Model file for the job. Use its own axes, mm. Face numbers are marked on the shaded views. Give positions to 0.01 mm unless a question says otherwise; leave off trailing zeros. Loops run counter-clockwise (first coordinate to the right, second up) from the corner with the lowest first, then second, coordinate; pieces in that order, holes last. Notation, with made-up numbers: M 66,-35.75 L 100,-35.75 A12 cw 100,-31.75 Z; hole C -7.75,-14.5 d9. An arc over 180 degrees is marked long. Answer in a Markdown table with one row per item.
```python
from build123d import *

# Parameters (mm, degrees)
F0_W     = 109
F0_H     = 109
F0_W_2   = 5
F0_H_2   = 5
F0_W_3   = 50
F0_H_3   = 50
F1_DEPTH = 2
F2_DEPTH = 5


with BuildPart() as f1:
    # F0 (on Top) → F1 (new body)
    with BuildSketch(Plane.XY):
        Rectangle(F0_W, F0_H)
        Polygon((-2.5, -52.5), (-52.5, -52.5), (-52.5, -2.5), (-52.5, 2.5), (-52.5, 52.5), (-2.5, 52.5), (2.5, 52.5), (52.5, 52.5), (52.5, 2.5), (52.5, -2.5), (52.5, -52.5), (2.5, -52.5), align=None, mode=Mode.SUBTRACT)
        Rectangle(F0_W_2, F0_H_2)
        with Locations((-27.5, 27.5)):
            Rectangle(F0_W_3, F0_H_3)
        with Locations((-27.5, -27.5)):
            Rectangle(F0_W_3, F0_H_3)
        with Locations((27.5, -27.5)):
            Rectangle(F0_W_3, F0_H_3)
        with Locations((27.5, 27.5)):
            Rectangle(F0_W_3, F0_H_3)
        with Locations((0, 27.5)):
            Rectangle(F0_W_2, F0_H_3)
        with Locations((27.5, 0)):
            Rectangle(F0_W_3, F0_H_2)
        with Locations((0, -27.5)):
            Rectangle(F0_W_2, F0_H_3)
        with Locations((-27.5, 0)):
            Rectangle(F0_W_3, F0_H_2)
    extrude(amount=F1_DEPTH)

    # F0 (on Top) → F2 (join)
    with BuildSketch(Plane.XY):
        Rectangle(F0_W, F0_H)
        Polygon((-2.5, -52.5), (-52.5, -52.5), (-52.5, -2.5), (-52.5, 2.5), (-52.5, 52.5), (-2.5, 52.5), (2.5, 52.5), (52.5, 52.5), (52.5, 2.5), (52.5, -2.5), (52.5, -52.5), (2.5, -52.5), align=None, mode=Mode.SUBTRACT)
        with Locations((0, -27.5)):
            Rectangle(F0_W_2, F0_H_3)
        with Locations((27.5, 0)):
            Rectangle(F0_W_3, F0_H_2)
        with Locations((-27.5, 0)):
            Rectangle(F0_W_3, F0_H_2)
        with Locations((0, 27.5)):
            Rectangle(F0_W_2, F0_H_3)
        Rectangle(F0_W_2, F0_H_2)
    extrude(amount=F2_DEPTH)


solid = f1.part
```
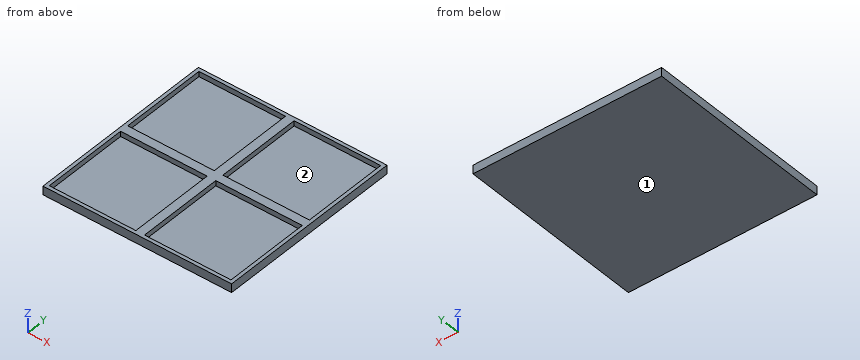
(1) Flat gauge pin, fed straight in: P1, Ø8, axis at x = 12.5, y = 20, coming from the +Z side. Where does the tip first touch, or does it go through?
Established:
| item | result |
|---|---|
| P1 | stops at z = 2 |
(2) Wall check: L1, parallel to Y at x = 45, z = 3.05; L2, parallel to Z at x = 11.5, y = -5.5. Give the ranges that are in metal, low to high.
Established:
| item | result |
|---|---|
| L1 | y = -54.5 to -52.5, -2.5 to 2.5, 52.5 to 54.5 |
| L2 | z = 0 to 2 |
(3) Saw through at B-B, the plane x = -6.5. Give the cut face in (y, z).
Established:
| item | result |
|---|---|
| outline | M -54.5,0 L 54.5,0 L 54.5,5 L 52.5,5 L 52.5,2 L 2.5,2 L 2.5,5 L -2.5,5 L -2.5,2 L -52.5,2 L -52.5,5 L -54.5,5 Z |
(4) Saw through at A-A, the plane z = 3.9. Give the cut face in (x, y).
Established:
| item | result |
|---|---|
| outline | M -54.5,-54.5 L 54.5,-54.5 L 54.5,54.5 L -54.5,54.5 Z; hole M -52.5,-52.5 L -2.5,-52.5 L -2.5,-2.5 L -52.5,-2.5 Z; hole M -52.5,2.5 L -2.5,2.5 L -2.5,52.5 L -52.5,52.5 Z; hole M 2.5,-52.5 L 52.5,-52.5 L 52.5,-2.5 L 2.5,-2.5 Z; hole M 2.5,2.5 L 52.5,2.5 L 52.5,52.5 L 2.5,52.5 Z |
(5) Mould opens along X. For the marked faces 1 and 2 say: pulls with the +X half, pulls with the -X half, needs draft (parallel to the pull), parting line crosses it, or undercut.
Established:
| item | result |
|---|---|
| face 1 | needs draft |
| face 2 | undercut |
